Can you work these out from the model? Positions are in its coordinate system, mm. A direction names the side the tool comes from. Coordinates: 2 decimals unless noted, no trailing zeros. Return JSON: item names as keys, results as strings. Group by question number.
1) Which directions (+Z, -Z, +X, -X, +Y, -Y) give clear straight access to the entire face, cutting with the end or side of a thin tool? Please do faces 1 (the face through (3.475, 0.306, 0.096)), 2 (the face through (6.16, -0.54, -2.44)).
2) For pin 1 Ø3 at (x, y) = (7.5, 2.5) entering from +Z; pin 2 Ø4 at (x, y) = (13, -0.5) entering from +Z; pin 3 Ø0.5 at (y, z) = (-1, -1.5) entering from -X, each with a flat end and sliding along its axis, tell me the tip position at first contact or that it passes through.
3) If I drill on line 1 along X through (y, z) = (-3, 2.25); line 2 along Y through (x, z) = (3, -0.25); line 3 along Y through (x, z) = (19, 0.75), over which ranges is the centre line in solid material (lowest first)?
```python
from build123d import *

# Parameters (mm, degrees)
FILLET1_R       = 0.2
FILLET2_R       = 0.5
HEX_2_DEPTH     = 2.5
THDSCHPAT_COUNT = 29
THDSCHPAT_PITCH = 0.779310345


with BuildPart() as part:
    # BodySke → Base-Revolve (revolve)
    with BuildSketch(Plane.XY):
        Polygon((0, 0), (0, 4.25), (5, 4.25), (5, 2.5), (29.555, 2.5), (30, 2.055), (30, 0), align=None)
    revolve(axis=Axis((-31.75, 0, 0), (1, 0, 0)))

    # Fillet1
    fillet1_edges = [part.edges().sort_by_distance(p)[0] for p in [
        (5, -2.5, 0),
    ]]
    fillet(fillet1_edges, radius=FILLET1_R)

    # Fillet2
    fillet2_edges = [part.edges().sort_by_distance(p)[0] for p in [
        (0, -4.25, 0),
    ]]
    fillet(fillet2_edges, radius=FILLET2_R)

    # Sketch2 → Hex-PreBroach (revolve, cut)
    with BuildSketch(Plane.XY):
        Polygon((0, 2.01), (2.5, 2.01), (3.660474041, 0), (0, 0), align=None)
    revolve(axis=Axis((0, 0, 0), (1, 0, 0)), mode=Mode.SUBTRACT)

    # Sketch3 → Hex 2 (cut)
    with BuildSketch(Plane(origin=(0, 0, 0), x_dir=(0, 0.5, 0.866025404), z_dir=(-1, 0, 0))):
        Polygon((1.160474041, 2.01), (-1.160474041, 2.01), (-2.320948082, 0), (-1.160474041, -2.01), (1.160474041, -2.01), (2.320948082, 0), align=None)
    extrude(amount=-HEX_2_DEPTH, mode=Mode.SUBTRACT)

    # ThdSchSke → ThreadSchematic (revolve, cut)
    with BuildSketch(Plane.XY):
        Polygon((7.4, -2.055), (7.088407645, -2.5), (7.088407645, -3.125), (7.711592355, -3.125), (7.711592355, -2.5), align=None)
    threadschematic = revolve(axis=Axis((-3.175, 0, 0), (1, 0, 0)), mode=Mode.SUBTRACT)

    # ThdSchPat: ThreadSchematic ×29
    with Locations(*[(i * THDSCHPAT_PITCH, 0, 0) for i in range(1, THDSCHPAT_COUNT)]):
        add(threadschematic, mode=Mode.SUBTRACT)


solid = part.part
```
Calculated:
{
 "1": {"face 1": "-X", "face 2": "+X"},
 "2": {"pin 1": "z = 2.28", "pin 2": "z = 2.5", "pin 3": "x = 2.5"},
 "3": {"line 1": "0 to 5", "line 2": "-4.24 to -1.12, 1.12 to 4.24", "line 3": "-2.05 to 2.05"}
}
